Work out the finished part from the listing and answer in its coordinate system (mm). Face numbers are marked on the shaded views. A direction names the side the tool comes from. Coordinates: 2 decimals unless noted, no trailing zeros. Order: outer loops, then holes, each group sorted by start corner. A loop starts at its lowest first (then second) coordinate and runs counter-clockwise, first axis right, second up. Notation, with made-up numbers: M -20,89.25 L -14,89.25 A22 cw -14,103.25 Z; hole C 49,20 d1. An arc over 180 degrees is marked long. Write item = value, one per line. Start each with the question number.
Q1. Straight lines are drawn through the part: line 1 along Y through (x, z) = (-9.75, 18.5) (3 decimals); line 2 along X through (y, z) = (-2.5, 16.5); line 3 along Z through (x, y) = (-6.35, -1.15). For each, find the intervals that lie inside material, in ascending order.
Q2. Find section A-A on z = 38.1. Give the vertices of the cut face in (x, y) (1 decimal), and give its area (3 significant figures).
Q3. Find section C-C on y = -5.5. Give the vertices of the cut face in (x, z), and give its area (3 significant figures).
Q4. Find section D-D on x = 9.25. Give the vertices of the cut face in (y, z) (3 decimals), and give its area (3 significant figures).
Q5. A tool of negligible diameter and unlimited length cuts with its end or side. For the marked faces 1, 2 and 3, from which of +Z, -Z, +X, -X, +Y, -Y can it reach the whole face along a straight path? Write none if from no direction.
Q6. Each of these flat-tipped pins is pushed along its axis until it touches: P1, Ø1, axis at x = -4, z = 65, coming from the +Y side; P2, Ø1, axis at x = 9.5, y = -3.5, coming from the +Z side; P3, Ø3.5, axis at y = -1, z = 50, coming from the +X side; P4, Ø4, axis at x = 3.5, z = 63.5, coming from the -Y side. Where does it stop, or does it pass through?
```python
from build123d import *

# Parameters (mm, degrees)
F1_DEPTH = 3.175
F3_DEPTH = 3.175
F5_DEPTH = 3.175
F8_D     = 3.175


with BuildPart() as f1:
    # F0 (on Front) → F1 (new body)
    with BuildSketch(Plane.XZ):
        Polygon((-12.7, 11.496929), (0, 0), (0, 73.66), (12.7, 76.746243), (12.7, 94.234135), (0, 97.856929), (-12.7, 97.856929), align=None)
    extrude(amount=F1_DEPTH)

    # F2 (on face) → F3 (join)
    with BuildSketch(Plane.XZ.offset(3.175)):
        Polygon((0, 97.856929), (-12.7, 97.856929), (-12.7, 73.66), (0, 73.66), (12.7, 76.746243), (12.7, 94.234135), align=None)
    extrude(amount=F3_DEPTH)

    # F4 (on face) → F5 (join)
    with BuildSketch(Plane(origin=(0, 0, 0), x_dir=(-1, 0, 0), z_dir=(0, 1, 0))):
        Polygon((-12.7, 76.746243), (0, 73.66), (12.7, 73.66), (12.7, 97.856929), (0, 97.856929), (-12.7, 94.234135), align=None)
    extrude(amount=F5_DEPTH)

    # F8 (through all)
    with Locations(Plane.XZ.offset(3.175)):
        with Locations((-6.35, 38.1)):
            Hole(F8_D / 2)


solid = f1.part
```
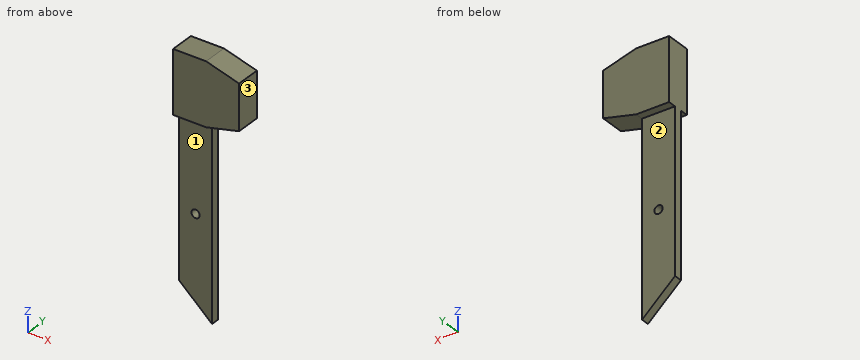
Findings below:
q1.line_1 = -3.175 to 0
q1.line_2 = -12.7 to 0
q1.line_3 = 5.75 to 36.51, 39.69 to 97.86
q2.outline = M -12.7,-3.2 L -7.9,-3.2 L -7.9,0 L -12.7,0 Z; M -4.8,-3.2 L 0,-3.2 L 0,0 L -4.8,0 Z
q2.area = 30.2 mm^2
q3.outline = M -12.7,73.66 L 0,73.66 L 12.7,76.75 L 12.7,94.23 L 0,97.86 L -12.7,97.86 Z
q3.area = 572 mm^2
q4.outline = M -6.35,75.908 L 3.175,75.908 L 3.175,95.218 L -6.35,95.218 Z
q4.area = 184 mm^2
q5.face_1 = -Z, +X, -X, -Y
q5.face_2 = -Z, +X, -X, +Y
q5.face_3 = +Z, -Z, +X, +Y, -Y
q6.P1 = 0
q6.P2 = 95.29
q6.P3 = 0
q6.P4 = through
